from build123d import *

# Parameters (mm, degrees)
HEXDIESKE_R  = 6.4443
HEXDIE_DEPTH = 0.8595


with BuildPart() as part:
    # BodySke → Body (revolve)
    with BuildSketch(Plane.XY, mode=Mode.PRIVATE) as body_sk:
        Polygon((4.500636445, 0), (5.785104, 0), (5.785104, 0.8595), (4.5, 0.8595), (4.5, 20.8595), (2.5, 20.8595), (2.5, 11.2595), (0, 11.2595), (0, -1.0505), (4.94, -1.0505), (4.94, -1.0475), (4.500636445, -0.2865), align=None)
    revolve(body_sk.sketch.rotate(Axis((0, 0, 0), (0, 1, 0)), 90), axis=Axis((0, 0, 0), (0, 1, 0)))

    # TapDriSke → TapDrill (revolve, cut)
    with BuildSketch(Plane.XY, mode=Mode.PRIVATE) as tapdrill_sk:
        Polygon((2.5, 6.2595), (2.5, 20.8595), (0, 20.8595), (0, 5.223966094), align=None)
    revolve(tapdrill_sk.sketch.rotate(Axis((0, 0, 0), (0, 1, 0)), 90), axis=Axis((0, 0, 0), (0, 1, 0)), mode=Mode.SUBTRACT)

    # EndChamferSke → EndChamfer (revolve, cut)
    with BuildSketch(Plane.XY, mode=Mode.PRIVATE) as endchamfer_sk:
        Polygon((3, 20.85696), (2.5, 20.506986267), (2.5, 21.1135), (3, 21.1135), align=None)
    revolve(endchamfer_sk.sketch.rotate(Axis((0, -2.54, 0), (0, 1, 0)), 90), axis=Axis((0, -2.54, 0), (0, 1, 0)), mode=Mode.SUBTRACT)

    # HexDieSke → HexDie (cut)
    with BuildSketch(Plane(origin=(0, 0.8595, 0), x_dir=(-1, 0, 0), z_dir=(0, 1, 0))):
        Circle(HEXDIESKE_R)
        Polygon((0, 6.414361491), (5.555, 3.207180745), (5.555, -3.207180745), (0, -6.414361491), (-5.555, -3.207180745), (-5.555, 3.207180745), align=None, mode=Mode.SUBTRACT)
    extrude(amount=-HEXDIE_DEPTH, mode=Mode.SUBTRACT)


solid = part.part
Build history of the part. All positions in model axes, mm. A direction names the side the tool comes from. Round coordinates to 2 decimals unless told otherwise and drop trailing zeros. Loops run counter-clockwise (first coordinate to the right, second up) from the corner with the lowest first, then second, coordinate; pieces in that order, holes last. Notation, with made-up numbers: (39.25, 28.25) -> (48.25, 28.25) arc R22 ccw to (48.25, 52.25) -> close; hole circle Ø7 at (-14.75, -11.5). An arc over 180 degrees is marked (long way). One line per item, written item: value. Start each with the question number.
Q1. Two-plate mould, pull along X, no slides. Class faces 1 (the face through (-5, 0, 1)), 2 (the face through (-5.02, 0.436, 2.876)), 3 (the face through (0.14, 5.29, -0.07)), 4 (the face through (5.555, 0.4, 0)): released by +X, released by -X, zero draft, split by the parting line, or undercut.
Q2. Drop flat-ended pins along their axis: pin 1 Ø5 at (x, y) = (3.5, 12) entering from -Z; pin 2 Ø5 at (x, y) = (-4.5, 13.5) entering from +Z; pin 3 Ø1 at (y, z) = (13.5, 3) entering from -X; pin 4 Ø3 at (x, y) = (-1, 1.5) entering from +Z. Give the stop position or say it passes through.
Q3. Probe line 1 along X through (y, z) = (16.75, 0); line 2 along Z through (x, y) = (-2, 18.25); line 3 along X through (y, z) = (9, 1.5). List the from-to ranges inside material, lowest first.
Q4. Cut at A-A on y = 19. List the corners of the cut face in (x, z), plus the area to 3 significant figures.
Q5. 3-axis set-ups, long thin cutter, end or side, ignore diameter. For faces 5 (the face through (-0.1, 13.3, 2.5)), 6 (the face through (2.8, 0.4, 4.8)): which of +Z, -Z, +X, -X, +Y, -Y reach the whole face in a straight line?
Computed:
1. face 1: zero draft
1. face 2: released by -X
1. face 3: undercut
1. face 4: released by +X
2. pin 1: z = -4.39
2. pin 2: z = 4.03
2. pin 3: x = -3.74
2. pin 4: z = 5.79
3. line 1: -4.5 to -2.5, 2.5 to 4.5
3. line 2: -4.03 to -1.5, 1.5 to 4.03
3. line 3: -4.24 to -2, 2 to 4.24
4. outline: circle Ø9 at (0, 0); hole circle Ø5 at (0, 0)
4. area: 44.0 mm²
5. face 5: +Y
5. face 6: +Z, +X, +Y, -Y
